```python
from build123d import *

# Parameters (mm, degrees)
SKETCH2_R                       = 10
BOSS_EXTRUDE1_DEPTH             = 13
F_11_0_11_M12X0_5_TAPPED_HOLE_D = 11
CHAMFER1_SIZE                   = 0.5
CUT_EXTRUDE8_START              = -7.895
SKETCH4_R                       = 6.15
CUT_EXTRUDE8_DEPTH              = 7.895
SKETCH5_R                       = 6.75
CUT_EXTRUDE9_DEPTH              = 1
SKETCH6_R                       = 19
SKETCH6_R_2                     = 6.15
BOSS_EXTRUDE2_DEPTH             = 3
CHAMFER2_SIZE                   = 0.5
M3_TAPPED_HOLE1_REACH           = 37.359
M3_TAPPED_HOLE1_BORE_R          = 1.25
F_3_8_3_8_DIAMETER_HOLE1_D      = 3.8
CIRPATTERN1_COUNT               = 3
CHAMFER4_SIZE                   = 0.5


with BuildPart() as part:
    # Sketch2 → Boss-Extrude1 (new body)
    with BuildSketch(Plane(origin=(0, 0, 0), x_dir=(0, 0, -1), z_dir=(1, 0, 0))):
        with Locations(Location((0, 0, 0), (0, 0, 180))):
            Circle(SKETCH2_R)
    extrude(amount=BOSS_EXTRUDE1_DEPTH)

    # Ø11.0 (11) M12x0.5 tapped hole (through all)
    with Locations(Plane(origin=(0, 0, 0), x_dir=(0, 0, -1), z_dir=(-1, 0, 0))):
        with Locations((0, 0)):
            Hole(F_11_0_11_M12X0_5_TAPPED_HOLE_D / 2)

    # Chamfer1
    chamfer1_edges = [part.edges().sort_by_distance(p)[0] for p in [
        (0, 0, -5.5),
    ]]
    chamfer(chamfer1_edges, length=CHAMFER1_SIZE)

    # Sketch4 → Cut-Extrude8 (cut)
    with BuildSketch(Plane(origin=(13, 0, 0), x_dir=(0, 0, -1), z_dir=(1, 0, 0)).offset(CUT_EXTRUDE8_START)):
        Circle(SKETCH4_R)
    extrude(amount=CUT_EXTRUDE8_DEPTH, mode=Mode.SUBTRACT)

    # Sketch5 → Cut-Extrude9 (cut)
    with BuildSketch(Plane(origin=(5.105, 0, 0), x_dir=(0, 0, -1), z_dir=(1, 0, 0))):
        Circle(SKETCH5_R)
    extrude(amount=CUT_EXTRUDE9_DEPTH, mode=Mode.SUBTRACT)

    # Sketch6 → Boss-Extrude2 (add)
    with BuildSketch(Plane(origin=(10, 0, 0), x_dir=(0, 0, -1), z_dir=(1, 0, 0))):
        Circle(SKETCH6_R)
        Circle(SKETCH6_R_2, mode=Mode.SUBTRACT)
    extrude(amount=BOSS_EXTRUDE2_DEPTH)

    # Chamfer2
    chamfer2_edges = [part.edges().sort_by_distance(p)[0] for p in [
        (13, 0, 6.15),
    ]]
    chamfer(chamfer2_edges, length=CHAMFER2_SIZE)

    # M3 Tapped Hole1 bore (on position points) → M3 Tapped Hole1 (cut, up to next)
    with BuildSketch(Plane(origin=(6.9465, 10, 0), x_dir=(0, 0, 1), z_dir=(0, 1, 0)), mode=Mode.PRIVATE) as m3_tapped_hole1_sk1:
        Circle(M3_TAPPED_HOLE1_BORE_R)
    m3_tapped_hole1_tool1 = extrude(m3_tapped_hole1_sk1.sketch, amount=-M3_TAPPED_HOLE1_REACH, mode=Mode.PRIVATE) & part.part
    add(m3_tapped_hole1_tool1.solids().sort_by_distance((6.9465, 10, 0))[0], mode=Mode.SUBTRACT)

    # Ø3.8 (3.8) Diameter Hole1 (through all)
    with Locations(Plane(origin=(13, -14, 0), x_dir=(0, 0, 1), z_dir=(1, 0, 0))):
        with Locations((0, 0)):
            f_3_8_3_8_diameter_hole1 = Hole(F_3_8_3_8_DIAMETER_HOLE1_D / 2)

    # CirPattern1: Ø3.8 (3.8) Diameter Hole1 ×3 about axis
    cirpattern1_axis = Axis((0, 0, 0), (1, 0, 0))
    for i in range(1, CIRPATTERN1_COUNT):
        add(f_3_8_3_8_diameter_hole1.rotate(cirpattern1_axis, i * 360 / CIRPATTERN1_COUNT), mode=Mode.SUBTRACT)

    # Chamfer4
    chamfer4_edges = [part.edges().sort_by_distance(p)[0] for p in [
        (0, 0, -10),
        (13, 0, 19),
        (10, 0, 19),
    ]]
    chamfer(chamfer4_edges, length=CHAMFER4_SIZE)


solid = part.part
```
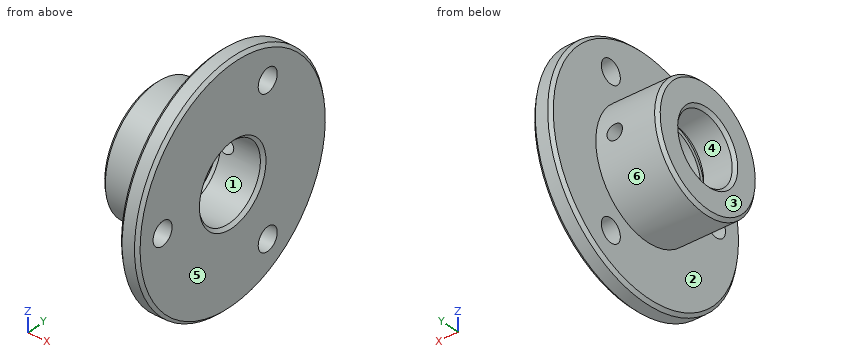
Work out the finished part from the listing and answer in its coordinate system (mm). Face numbers are marked on the shaded views. A direction names the side the tool comes from. Round coordinates to 2 decimals unless told otherwise and drop trailing zeros. Loops run counter-clockwise (first coordinate to the right, second up) from the corner with the lowest first, then second, coordinate; pieces in that order, holes last. Notation, with made-up numbers: M 40.25,-0.75 L 79.25,-0.75 A7 cw 79.25,9.25 Z; hole C -2.5,21.5 d1. An arc over 180 degrees is marked long. One line per question, with ' | ' between items.
Q1. Each of these flat-tipped pins is pushed along its axis until it touches: pin 1 Ø4 at (x, z) = (11, -6) entering from +Y; pin 2 Ø1.5 at (y, z) = (-7, -6.5) entering from -X; pin 3 Ø6 at (y, z) = (10.5, 8) entering from -X; pin 4 Ø7.5 at (y, z) = (0, 0) entering from +X. Where does it stop, or does it pass through?
Conclusion:
pin 1: stops at y = 18.57 | pin 2: stops at x = 0 | pin 3: stops at x = 10 | pin 4: passes through
Q2. Find section C-C, the plane x = 8.75. Give the vertices of the cut face in (y, z).
Conclusion:
outline: C 0,0 d20; hole C 0,0 d12.3
Q3. Find section B-B, the plane z = 0. State how many separate pieces and enclosed holes the cut face has, then the cut area to 3 significant figures.
Conclusion:
separate pieces: 4 | enclosed holes: 0 | area: 138 mm2
Q4. A tool of negligible diameter and unlimited length cuts with its end or side. For the marked faces 1, 2 and 3, from which of +Z, -Z, +X, -X, +Y, -Y can it reach the whole face along a straight path? Write none if from no direction.
Conclusion:
face 1: +X | face 2: -X | face 3: +Z, -Z, -X, +Y, -Y
Q5. The mould has two halves that part along Z. Classify the marked faces 4, 5 and 6: +Z half, -Z half, draft (parallel to the pull), parting line (faces both ways), or undercut.
Conclusion:
face 4: undercut | face 5: draft | face 6: parting line
Q6. Find section D-D, the plane x = 3.5. Give the vertices of the cut face in (y, z).
Conclusion:
outline: C 0,0 d20; hole C 0,0 d11
Q7. Consider line 1 along Y through (x, z) = (5.6, 0); line 2 along X through (y, z) = (9, 6); line 3 along Z through (x, y) = (5.5, 5). Determine where each line is inside the solid, lowest interval first. Write a range as from..to.
Conclusion:
line 1: y = -10..-6.75, 6.75..10 | line 2: x = 10..13 | line 3: z = -8.66..-4.53, 4.53..8.66
